Geometry check sheet. Reference: drawing and pictorial views, mm from the part's lowest x, y, z. A direction names the side the tool comes from. Give positions to 0.01 mm unless a question says otherwise; leave off trailing zeros. Write each loop counter-clockwise with the first axis right and the second up, starting at its lowest first coordinate (ties: lowest second). Pieces come first, ordered by that corner, then holes. Notation, with made-up numbers: (7, 74.25) -> (26, 74.25) arc R13 cw to (26, 88.25) -> close; hole circle Ø5 at (27, 22.5). An arc over 180 degrees is marked (long way). Return JSON: item names as keys, results as strings.
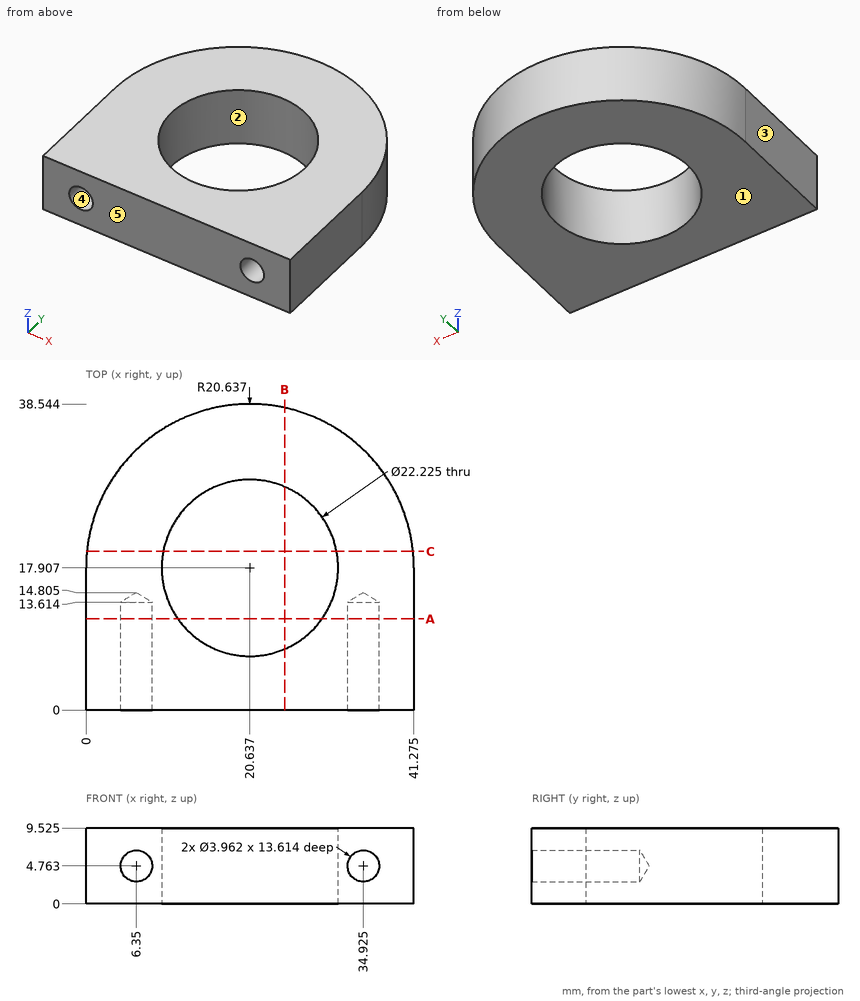
(1) Depth check by flat-ended pin: pin 1 Ø1.5 at (x, z) = (5, 7) entering from +Y; pin 2 Ø3 at (x, z) = (6.35, 4.76) entering from +Y (1 decimal). Enter the tip coordinate at first touch or a pass-through.
Reply:
{"pin 1": "y = 32.2", "pin 2": "y = 34.1"}
(2) Cross-section at B-B on x = 25. Enter the section's corners in (y, z) (1 decimal).
Reply:
{"outline": "(0, 0) -> (7.7, 0) -> (7.7, 9.5) -> (0, 9.5) -> close; (28.1, 0) -> (38.1, 0) -> (38.1, 9.5) -> (28.1, 9.5) -> close"}
(3) Release check for a two-part mould opening along X. For the marked faces 1, 2 and 3 record: pulls with the +X half, pulls with the -X half, needs draft (parallel to the pull), parting line crosses it, or undercut.
Reply:
{"face 1": "needs draft", "face 2": "undercut", "face 3": "pulls with the -X half"}
(4) Cross-section at C-C on y = 20. Enter the section's corners in (x, z) (1 decimal).
Reply:
{"outline": "(0.1, 0) -> (9.7, 0) -> (9.7, 9.5) -> (0.1, 9.5) -> close; (31.6, 0) -> (41.2, 0) -> (41.2, 9.5) -> (31.6, 9.5) -> close"}
(5) Set-up check for the marked faces 4 and 5: record each of +Z, -Z, +X, -X, +Y, -Y from which the full face is reachable in a straight line by a thin tool's end or side.
Reply:
{"face 4": "-Y", "face 5": "+Z, -Z, +X, -X, -Y"}
(6) Cross-section at A-A on y = 11.5. State how many separate pieces and enclosed holes the cut face has.
Reply:
{"separate pieces": "2", "enclosed holes": "2"}
(7) Thickness scan on L1, parallel to Z at x = 35, y = 8 (1 decimal); L2, parallel to X at y = 11, z = 5.5 (1 decimal); L3, parallel to X at y = 3, z = 5 (1 decimal). Record the ranges inside material, lowest first.
Reply:
{"L1": "0 to 2.8, 6.7 to 9.5", "L2": "0 to 4.5, 8.2 to 11.9, 29.3 to 33.1, 36.8 to 41.3", "L3": "0 to 4.4, 8.3 to 33, 36.9 to 41.3"}
